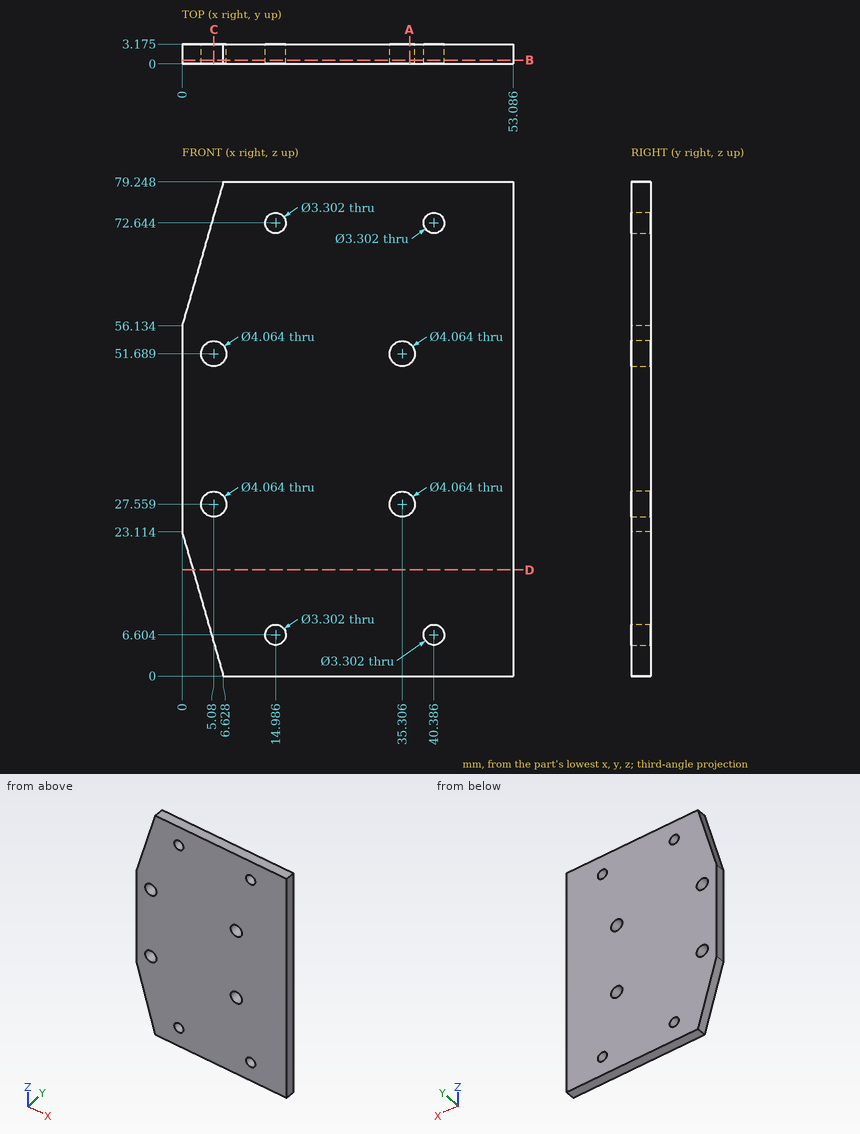
For this review, use the dimensioned drawing (mm, ordinates from the lowest corner) and the shaded views. Coordinates: 2 decimals unless noted, no trailing zeros. Write each loop counter-clockwise with the first axis right and the second up, starting at its lowest first coordinate (ties: lowest second). Pieces come first, ordered by that corner, then holes. Notation, with made-up numbers: (-9, 24) - (31, 24) arc R5 cw to (31, 29) - close; hole circle Ø7 at (-2, -6.5). An arc over 180 degrees is marked (long way). Answer as a JSON object with one key per item and string values. Group by question number.
1. Add section C-C (x = 5.08). Give the boundary of the cut face in (y, z) (3 decimals).
2. Clearance check with a flat-ended pin moving along its axis: pin 1 Ø2.5 at (x, z) = (40.386, 72.644) entering from -Y. State where the tip first meets the part, or that it passes through.
3. Add section B-B (y = 0.6). Give the number of separate pieces and of enclosed holes in the cut face, plus the area to 3 significant figures.
4. To check wall thickness, follow probe 1 along X at (y, z) = (1.65, 73.5) (1 decimal); probe 2 along X at (y, z) = (0.85, 8) (1 decimal); probe 3 along Z at (x, y) = (35, 3). State the ranges of each line that lie inside material, in increasing order.
5. Add section D-D (z = 17). Give the boundary of the cut face in (x, y) (1 decimal).
6. Add section A-A (x = 36.5). Give the boundary of the cut face in (y, z) (1 decimal).
Findings:
{
 "1": {"outline": "(0, 5.398) - (3.175, 5.398) - (3.175, 25.527) - (0, 25.527) - close; (0, 29.591) - (3.175, 29.591) - (3.175, 49.657) - (0, 49.657) - close; (0, 53.721) - (3.175, 53.721) - (3.175, 73.85) - (0, 73.85) - close"},
 "2": {"pin 1": "through"},
 "3": {"separate pieces": "1", "enclosed holes": "8", "area": "3,970 mm²"},
 "4": {"probe 1": "5 to 13.6, 16.4 to 39, 41.8 to 53.1", "probe 2": "4.3 to 14.1, 15.9 to 39.5, 41.3 to 53.1", "probe 3": "0 to 25.55, 29.57 to 49.68, 53.7 to 79.25"},
 "5": {"outline": "(1.8, 0) - (53.1, 0) - (53.1, 3.2) - (1.8, 3.2) - close"},
 "6": {"outline": "(0, 0) - (3.2, 0) - (3.2, 25.9) - (0, 25.9) - close; (0, 29.2) - (3.2, 29.2) - (3.2, 50) - (0, 50) - close; (0, 53.3) - (3.2, 53.3) - (3.2, 79.2) - (0, 79.2) - close"}
}
